Design review of the part shown in the three views and the two pictorial views. Dimensions are in mm from the part's minimum x, y and z. Coordinates: 2 decimals unless noted, no trailing zeros. Write each loop counter-clockwise with the first axis right and the second up, starting at its lowest first coordinate (ties: lowest second). Pieces come first, ordered by that corner, then holes. Notation, with made-up numbers: (5, 22) -> (62, 22) arc R28 cw to (62, 57) -> close; hole circle Ø8 at (17, 72.5). An arc over 180 degrees is marked (long way). Write each question's results on one line, items separated by ' | '.
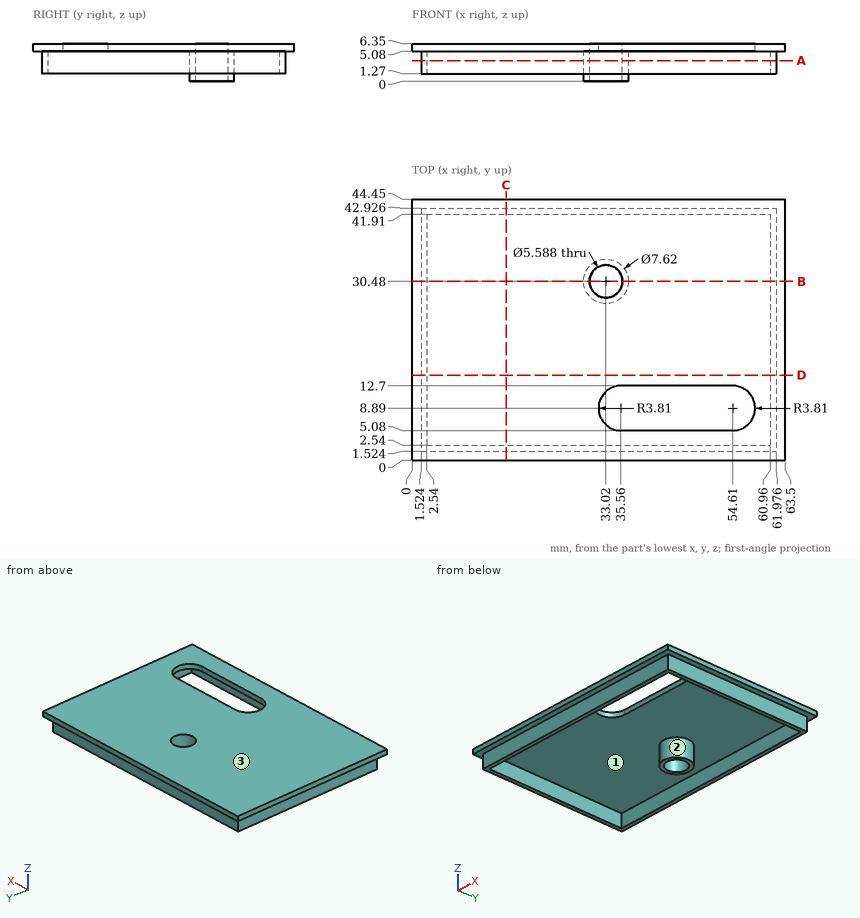
Q1. Clearance check with flat-ended pins moving along their axes: P1, Ø3, axis at y = 26.5, z = 3.5, coming from the +X side; P2, Ø3, axis at x = 18.5, z = 3, coming from the +Y side; P3, Ø3, axis at x = 47, z = 3, coming from the -Y side. State where each tip first meets the part, or that it passes through.
Solution:
P1: x = 61.98 | P2: y = 42.93 | P3: y = 1.52
Q2. Add section A-A (z = 3.5). Write out the cut boundary in (x, y).
Solution:
outline: (1.52, 1.52) -> (61.98, 1.52) -> (61.98, 42.93) -> (1.52, 42.93) -> close; circle Ø7.62 at (33.02, 30.48); hole (2.54, 2.54) -> (60.96, 2.54) -> (60.96, 41.91) -> (2.54, 41.91) -> close; hole circle Ø5.59 at (33.02, 30.48)
Q3. Add section B-B (y = 30.48). Write out the cut boundary in (x, z), plus the area to 3 significant figures.
Solution:
outline: (0, 5.08) -> (1.52, 5.08) -> (1.52, 1.27) -> (2.54, 1.27) -> (2.54, 5.08) -> (29.21, 5.08) -> (29.21, 0) -> (30.23, 0) -> (30.23, 6.35) -> (0, 6.35) -> close; (35.81, 0) -> (36.83, 0) -> (36.83, 5.08) -> (60.96, 5.08) -> (60.96, 1.27) -> (61.98, 1.27) -> (61.98, 5.08) -> (63.5, 5.08) -> (63.5, 6.35) -> (35.81, 6.35) -> close | area: 91.6 mm²
Q4. Draft analysis for pull direction Y (two halves, no side actions). For the marked faces 1, 2 and 3, state which applies: pulls with the +Y half, pulls with the -Y half, needs draft (parallel to the pull), parting line crosses it, or undercut.
Solution:
face 1: undercut | face 2: undercut | face 3: needs draft
Q5. Add section C-C (x = 16). Write out the cut boundary in (y, z), plus the area to 3 significant figures.
Solution:
outline: (0, 5.08) -> (1.52, 5.08) -> (1.52, 1.27) -> (2.54, 1.27) -> (2.54, 5.08) -> (41.91, 5.08) -> (41.91, 1.27) -> (42.93, 1.27) -> (42.93, 5.08) -> (44.45, 5.08) -> (44.45, 6.35) -> (0, 6.35) -> close | area: 64.2 mm²
Q6. Add section D-D (y = 14.5). Write out the cut boundary in (x, z).
Solution:
outline: (0, 5.08) -> (1.52, 5.08) -> (1.52, 1.27) -> (2.54, 1.27) -> (2.54, 5.08) -> (60.96, 5.08) -> (60.96, 1.27) -> (61.98, 1.27) -> (61.98, 5.08) -> (63.5, 5.08) -> (63.5, 6.35) -> (0, 6.35) -> close
Q7. For line 1 (Y direction, x = 33.02, z = 4); line 2 (X direction, y = 30.48, z = 5); line 3 (Y direction, x = 13.5, z = 5), list the stretches that pass through material, from the lowest coordinate up. Write a range as from..to.
Solution:
line 1: 1.52..2.54, 26.67..27.69, 33.27..34.29, 41.91..42.93 | line 2: 1.52..2.54, 29.21..30.23, 35.81..36.83, 60.96..61.98 | line 3: 1.52..2.54, 41.91..42.93
